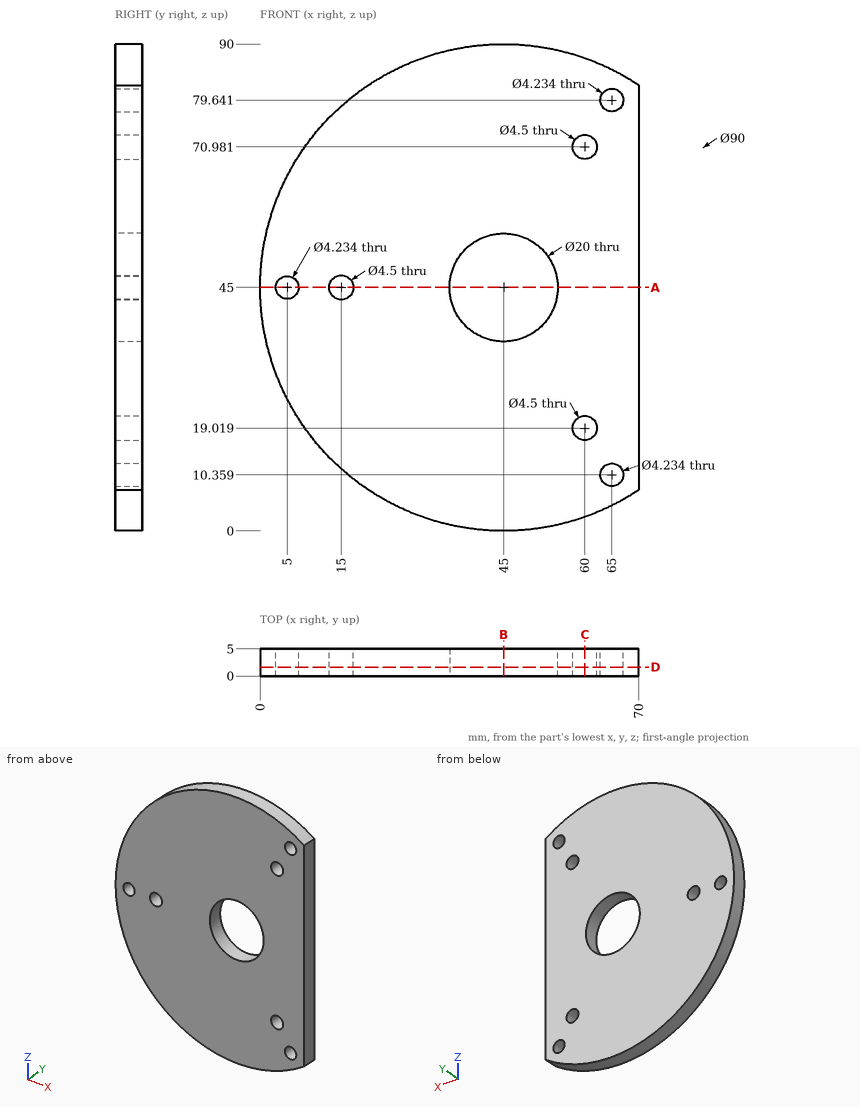
Geometry check sheet. Reference: drawing and pictorial views, mm from the part's lowest x, y, z. Round coordinates to 2 decimals unless told otherwise and drop trailing zeros. Loops run counter-clockwise (first coordinate to the right, second up) from the corner with the lowest first, then second, coordinate; pieces in that order, holes last. Notation, with made-up numbers: (6, -12) -> (44, -12) arc R20 cw to (44, 15) -> close; hole circle Ø3 at (-8, 5). An arc over 180 degrees is marked (long way). Use a Markdown table: item, result.
(1) Sectioned sample at D-D (y = 1.65). Enter the section's corners in (x, z).
Calculated:
| item | result |
|---|---|
| outline | (70, 7.58) -> (70, 82.42) arc R45 ccw (long way) to start; hole circle Ø4.23 at (5, 45); hole circle Ø4.5 at (15, 45); hole circle Ø20 at (45, 45); hole circle Ø4.5 at (60, 19.02); hole circle Ø4.5 at (60, 70.98); hole circle Ø4.23 at (65, 10.36); hole circle Ø4.23 at (65, 79.64) |
(2) Scan lines: probe 1 along X at (y, z) = (3.45, 45); probe 2 along Z at (x, y) = (45, 1.35); probe 3 along Z at (x, y) = (65, 1.2). Record each from-to range of solid material in increasing order.
Calculated:
| item | result |
|---|---|
| probe 1 | 0 to 2.88, 7.12 to 12.75, 17.25 to 35, 55 to 70 |
| probe 2 | 0 to 35, 55 to 90 |
| probe 3 | 4.69 to 8.24, 12.48 to 77.52, 81.76 to 85.31 |
(3) Sectioned sample at C-C (x = 60). Enter the section's corners in (y, z).
Calculated:
| item | result |
|---|---|
| outline | (0, 2.57) -> (5, 2.57) -> (5, 16.77) -> (0, 16.77) -> close; (0, 21.27) -> (5, 21.27) -> (5, 68.73) -> (0, 68.73) -> close; (0, 73.23) -> (5, 73.23) -> (5, 87.43) -> (0, 87.43) -> close |
(4) Go/stop test with flat-tipped pins: P1, Ø4, axis at x = 65, z = 79.641, coming from the +Y side; P2, Ø5, axis at x = 60, z = 70.98, coming from the -Y side; P3, Ø2, axis at x = 25.5, y = 4, coming from the +Z side. Record where each tip stops, or that it passes through.
Calculated:
| item | result |
|---|---|
| P1 | through |
| P2 | y = 0 |
| P3 | z = 86.02 |
(5) Sectioned sample at A-A (z = 45). Enter the section's corners in (x, y).
Calculated:
| item | result |
|---|---|
| outline | (0, 0) -> (2.88, 0) -> (2.88, 5) -> (0, 5) -> close; (7.12, 0) -> (12.75, 0) -> (12.75, 5) -> (7.12, 5) -> close; (17.25, 0) -> (35, 0) -> (35, 5) -> (17.25, 5) -> close; (55, 0) -> (70, 0) -> (70, 5) -> (55, 5) -> close |
(6) Sectioned sample at B-B (x = 45). Enter the section's corners in (y, z), then the cut area to 3 significant figures.
Calculated:
| item | result |
|---|---|
| outline | (0, 0) -> (5, 0) -> (5, 35) -> (0, 35) -> close; (0, 55) -> (5, 55) -> (5, 90) -> (0, 90) -> close |
| area | 350 mm² |
